from build123d import *

# Parameters (mm, degrees)
F0_R     = 19.05
F1_DEPTH = 3.175
F2_D     = 3.81
F3_D     = 3.81


with BuildPart() as f1:
    # F0 (on Front) → F1 (new body, symmetric)
    with BuildSketch(Plane.XZ):
        Circle(F0_R)
    extrude(amount=F1_DEPTH, both=True)

    # F2 (through all)
    with Locations(Plane.XZ):
        with Locations((15.24, 0), (-15.24, 0)):
            Hole(F2_D / 2)

    # F3 (through all)
    with Locations(Plane(origin=(0, 0, 0), x_dir=(1, 0, 0), z_dir=(0, 1, 0))):
        with Locations((-15.24, 0), (15.24, 0)):
            Hole(F3_D / 2)


solid = f1.part
Read the model definition and answer for the solid it produces. Units are mm, in the model's axes. Give positions to 0.01 mm unless a question says otherwise; leave off trailing zeros. Write each loop counter-clockwise with the first axis right and the second up, starting at its lowest first coordinate (ties: lowest second). Pieces come first, ordered by that corner, then holes. Notation, with made-up numbers: (87, 33.5) - (115, 33.5) arc R27 ccw to (115, 51.5) - close; hole circle Ø3 at (53.5, 46.25). An arc over 180 degrees is marked (long way). Use CSV: the item, a comma, the result in double quotes. Start each with the question number.
(1) Find section A-A (z = 0). Give the vertices of the cut face in (x, y) (3 decimals), plus the area to 3 significant figures.
(2) Find section C-C (y = -2). Give the vertices of the cut face in (x, z) (3 decimals), plus the area to 3 significant figures.
(3) Find section D-D (z = 9.5). Give the vertices of the cut face in (x, y) (3 decimals), plus the area to 3 significant figures.
(4) Find section B-B (x = -15.24). Give the vertices of the cut face in (y, z) (3 decimals).
(5) Given P1, Ø5, axis at x = -15.24, z = 0, coming from the +Y side (3 decimals); P2, Ø1, axis at x = -6, y = -0.5, coming from the -Z side; P3, Ø3, axis at y = 1.5, z = 11, coming from the -X side; P4, Ø3, axis at x = 15.24, z = 0, coming from the +Y side, each flat-ended and moving along its own axis, determine where each tip first touches the part or whether it passes through.
(6) Determine the mould class of faces 1 (the cylindrical face through (16.64, 0.04, 1.29)), 2 (the cylindrical face through (-15.12, -0.04, -11.59)), 3 (the flat face through (0, 3.175, 0)) for opening direction X: +X half, -X half, draft (parallel to the pull), parting line (faces both ways), or undercut.
(7) Consider line 1 along Z through (x, y) = (-15.5, 0); line 2 along Z through (x, y) = (15.24, -0.5) (3 decimals); line 3 along Z through (x, y) = (11.5, 1.25). Determine where each line is inside the solid, lowest interval first.
Findings below:
1,outline,"(-19.05, -3.175) - (-17.145, -3.175) - (-17.145, 3.175) - (-19.05, 3.175) - close; (-13.335, -3.175) - (13.335, -3.175) - (13.335, 3.175) - (-13.335, 3.175) - close; (17.145, -3.175) - (19.05, -3.175) - (19.05, 3.175) - (17.145, 3.175) - close"
1,area,"194 mm2"
2,outline,"circle Ø38.1 at (0, 0); hole circle Ø3.81 at (-15.24, 0); hole circle Ø3.81 at (15.24, 0)"
2,area,"1,120 mm2"
3,outline,"(-16.512, -3.175) - (16.512, -3.175) - (16.512, 3.175) - (-16.512, 3.175) - close"
3,area,"210 mm2"
4,outline,"(-3.175, -11.43) - (3.175, -11.43) - (3.175, -1.905) - (-3.175, -1.905) - close; (-3.175, 1.905) - (3.175, 1.905) - (3.175, 11.43) - (-3.175, 11.43) - close"
5,P1,"y = 3.175"
5,P2,"z = -18.24"
5,P3,"x = -16.51"
5,P4,"through"
6,face 1,"undercut"
6,face 2,"parting line"
6,face 3,"draft"
7,line 1,"-11.07 to -1.89, 1.89 to 11.07"
7,line 2,"-11.43 to -1.905, 1.905 to 11.43"
7,line 3,"-15.19 to 15.19"
